Can you work these out from the model? Positions are in its coordinate system, mm. Face numbers are marked on the shaded views. A direction names the side the tool comes from. Give positions to 0.01 mm unless a question says otherwise; leave off trailing zeros. Loops run counter-clockwise (first coordinate to the right, second up) from the corner with the lowest first, then second, coordinate; pieces in that order, holes last. Notation, with made-up numbers: (-6, -13.5) - (51, -13.5) arc R26 cw to (51, 9.5) - close; hole circle Ø2 at (-18.5, 64.25). An arc over 180 degrees is marked (long way). Answer as a JSON object with one key per item and string values.
```python
from build123d import *

# Parameters (mm, degrees)
SKETCH1_R           = 16
BOSS_EXTRUDE1_DEPTH = 5
SKETCH2_R           = 10
BOSS_EXTRUDE2_DEPTH = 24
SKETCH4_OUTSIDE_W   = 44.75
SKETCH4_OUTSIDE_H   = 44.75
SKETCH4_OUTSIDE_W_2 = 24
SKETCH4_OUTSIDE_H_2 = 17.6
CUT_EXTRUDE1_DEPTH  = 9
SKETCH5_R           = 14
BOSS_EXTRUDE3_DEPTH = 19.6


with BuildPart() as part:
    # Sketch1 → Boss-Extrude1 (new body)
    with BuildSketch(Plane.XY):
        Circle(SKETCH1_R)
    extrude(amount=BOSS_EXTRUDE1_DEPTH)

    # Sketch2 → Boss-Extrude2 (add)
    with BuildSketch(Plane.XY.offset(5)):
        Circle(SKETCH2_R)
    extrude(amount=BOSS_EXTRUDE2_DEPTH)

    # Sketch4 outside → Cut-Extrude1 (cut)
    with BuildSketch(Plane.XY.offset(7)):
        Rectangle(SKETCH4_OUTSIDE_W, SKETCH4_OUTSIDE_H)
        Rectangle(SKETCH4_OUTSIDE_W_2, SKETCH4_OUTSIDE_H_2, mode=Mode.SUBTRACT)
    extrude(amount=CUT_EXTRUDE1_DEPTH, mode=Mode.SUBTRACT)

    # Sketch5 → Boss-Extrude3 (add)
    with BuildSketch(Plane.XY.offset(18)):
        Circle(SKETCH5_R)
    extrude(amount=BOSS_EXTRUDE3_DEPTH)


solid = part.part
```
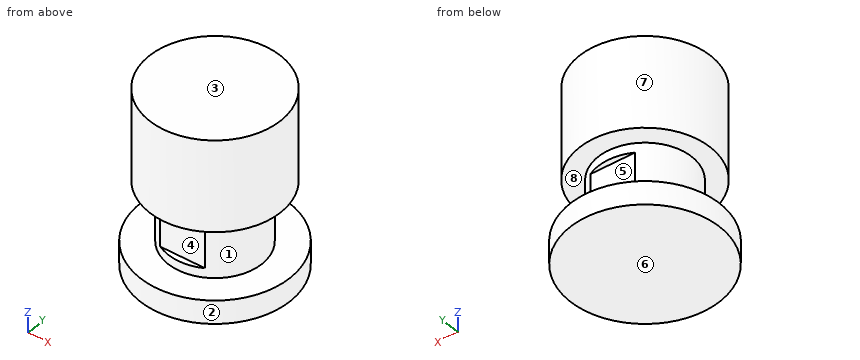
1) Imagine slicing it at C-C on y = 9.5. Write out the boundary of the cut face in (x, z).
Check sheet entries:
{"outline": "(-12.87, 0) - (12.87, 0) - (12.87, 5) - (3.12, 5) - (3.12, 7) - (-3.12, 7) - (-3.12, 5) - (-12.87, 5) - close; (-10.28, 18) - (-3.12, 18) - (-3.12, 16) - (3.12, 16) - (3.12, 18) - (10.28, 18) - (10.28, 37.6) - (-10.28, 37.6) - close"}
2) Imagine slicing it at B-B on x = 0. Write out the boundary of the cut face in (y, z), and give its area (3 significant figures).
Check sheet entries:
{"outline": "(-16, 0) - (16, 0) - (16, 5) - (10, 5) - (10, 7) - (8.8, 7) - (8.8, 16) - (10, 16) - (10, 18) - (14, 18) - (14, 37.6) - (-14, 37.6) - (-14, 18) - (-10, 18) - (-10, 16) - (-8.8, 16) - (-8.8, 7) - (-10, 7) - (-10, 5) - (-16, 5) - close", "area": "947 mm2"}
3) Imagine slicing it at D-D on z = 35.5. Write out the boundary of the cut face in (x, y), and give its area (3 significant figures).
Check sheet entries:
{"outline": "circle Ø28 at (0, 0)", "area": "616 mm2"}
4) Which directions (+Z, -Z, +X, -X, +Y, -Y) give clear straight access to the entire face, cutting with the end or side of a thin tool? Please do the marked faces 1, 2, 3, 4 and 5.
Check sheet entries:
{"face 1": "none", "face 2": "+Z, -Z", "face 3": "+Z, +X, -X, +Y, -Y", "face 4": "+X, -X, -Y", "face 5": "+X, -X, +Y"}
5) I need wall thicknesses on L1, parallel to Z at x = 0, y = -13; L2, parallel to Z at x = -4, y = -13.5; L3, parallel to Y at x = -2.5, z = 9.5. Which ranges of each line are inside material? Lowest first, please.
Check sheet entries:
{"L1": "0 to 5, 18 to 37.6", "L2": "0 to 5", "L3": "-8.8 to 8.8"}
6) I'm going to push flat-ended pins straight in: P1, Ø10, axis at x = 3, z = 33.5, coming from the +Y side; P2, Ø4, axis at x = 2, z = 31, coming from the -Y side; P3, Ø5, axis at y = 7, z = 17, coming from the +X side; P4, Ø1, axis at x = 1.5, y = 9, coming from the -Z side. Where does each tip first touch, or does it pass through?
Check sheet entries:
{"P1": "y = 14", "P2": "y = -14", "P3": "x = 13.18", "P4": "z = 0"}
7) Imagine slicing it at A-A on y = 0. Write out the boundary of the cut face in (x, z), and give its area (3 significant figures).
Check sheet entries:
{"outline": "(-16, 0) - (16, 0) - (16, 5) - (10, 5) - (10, 18) - (14, 18) - (14, 37.6) - (-14, 37.6) - (-14, 18) - (-10, 18) - (-10, 5) - (-16, 5) - close", "area": "969 mm2"}
8) If we mould it in two halves opening along Z, with no side actions, what happens to the marked faces 6, 7 and 8? For each: released by +Z, released by -Z, zero draft, split by the parting line, or undercut.
Check sheet entries:
{"face 6": "released by -Z", "face 7": "zero draft", "face 8": "undercut"}
